from build123d import *

# Parameters (mm, degrees)
SKETCH1_W           = 5.2
SKETCH1_H           = 32
SKETCH1_R           = 1.3
BOSS_EXTRUDE1_DEPTH = 2.8
SKETCH2_W           = 32
SKETCH2_H           = 10
BOSS_EXTRUDE2_DEPTH = 7.9
SKETCH3_W           = 3.95
SKETCH3_H           = 32
CUT_EXTRUDE1_DEPTH  = 7.2
FILLET1_R           = 2


with BuildPart() as part:
    # Sketch1 → Boss-Extrude1 (new body)
    with BuildSketch(Plane(origin=(0, 0, 0), x_dir=(1, 0, 0), z_dir=(0, 1, 0))):
        Rectangle(SKETCH1_W, SKETCH1_H)
        with Locations((0, -8.5)):
            Circle(SKETCH1_R, mode=Mode.SUBTRACT)
        with Locations((0, 8.5)):
            Circle(SKETCH1_R, mode=Mode.SUBTRACT)
    extrude(amount=BOSS_EXTRUDE1_DEPTH)

    # Sketch2 → Boss-Extrude2 (add)
    with BuildSketch(Plane(origin=(2.6, 0, 0), x_dir=(0, 0, -1), z_dir=(1, 0, 0))):
        with Locations((0, 5)):
            Rectangle(SKETCH2_W, SKETCH2_H)
    extrude(amount=BOSS_EXTRUDE2_DEPTH)

    # Sketch3 → Cut-Extrude1 (cut)
    with BuildSketch(Plane(origin=(0, 10, 0), x_dir=(1, 0, 0), z_dir=(0, 1, 0))):
        with Locations((4.575, 0)):
            Rectangle(SKETCH3_W, SKETCH3_H)
    extrude(amount=-CUT_EXTRUDE1_DEPTH, mode=Mode.SUBTRACT)

    # Fillet1
    fillet1_edges = [part.edges().sort_by_distance(p)[0] for p in [
        (6.55, 2.8, 0),
    ]]
    fillet(fillet1_edges, radius=FILLET1_R)


solid = part.part
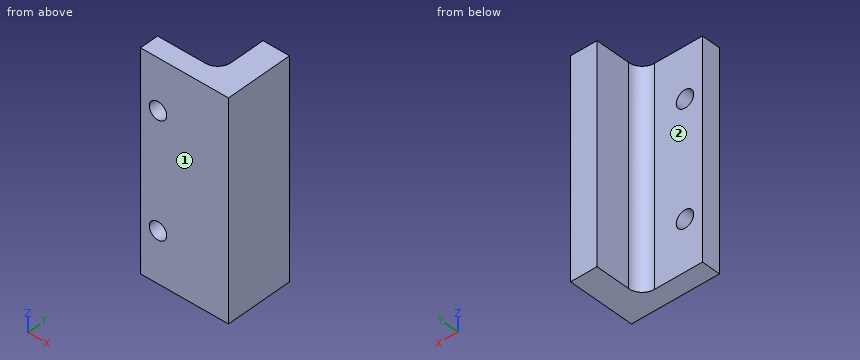
Can you work these out from the model? Positions are in its coordinate system, mm. Face numbers are marked on the shaded views. A direction names the side the tool comes from. Round coordinates to 2 decimals unless told otherwise and drop trailing zeros. Loops run counter-clockwise (first coordinate to the right, second up) from the corner with the lowest first, then second, coordinate; pieces in that order, holes last. Notation, with made-up numbers: (28, 17) - (78, 17) arc R7 ccw to (78, 24) - close; hole circle Ø2 at (-26, -8). An arc over 180 degrees is marked (long way). Write item = value, one per line. Start each with the question number.
(1) For P1, Ø3, axis at y = 9, z = 9.5, coming from the -X side; P2, Ø4, axis at y = 6.5, z = -5.5, coming from the -X side; P3, Ø5, axis at x = 5, z = -9, coming from the +Y side; P4, Ø5.5, axis at x = 2.5, z = -6, coming from the +Y side, each with a flat end and sliding along its axis, tell me the tip position at first contact or that it passes through.
(2) If we section it at D-D (z = -1): Please give me the cut outline in (x, y).
(3) If we section it at C-C (y = 1): Please give me the cut outline in (x, z).
(4) If we section it at B-B (x = 0): Please give me the cut outline in (y, z), and give its area (3 significant figures).
(5) If we section it at A-A (z = 8.5): Please give me the cut outline in (x, y), and give its area (3 significant figures).
(6) If I drill on probe 1 along Z at (x, y) = (0, 1.5); probe 2 along X at (y, z) = (1.6, 8.5); probe 3 along Y at (x, z) = (4.5, 5), over which ranges is the centre line in solid material (lowest first)? Write a range as [from, to].
(7) For the marked faces 1 and 2, which set-ups out of +Z, -Z, +X, -X, +Y, -Y let a thin tool reach every point of the face, with its end or its side?
Ans:
q1.P1 = 6.55
q1.P2 = 6.53
q1.P3 = 10
q1.P4 = 2.93
q2.outline = (-2.6, 0) - (10.5, 0) - (10.5, 10) - (6.55, 10) - (6.55, 4.8) arc R2 cw to (4.55, 2.8) - (-2.6, 2.8) - close
q3.outline = (-2.6, -16) - (10.5, -16) - (10.5, 16) - (-2.6, 16) - close; hole circle Ø2.6 at (0, -8.5); hole circle Ø2.6 at (0, 8.5)
q4.outline = (0, -16) - (2.8, -16) - (2.8, -9.8) - (0, -9.8) - close; (0, -7.2) - (2.8, -7.2) - (2.8, 7.2) - (0, 7.2) - close; (0, 9.8) - (2.8, 9.8) - (2.8, 16) - (0, 16) - close
q4.area = 75.0 mm²
q5.outline = (-2.6, 0) - (-1.3, 0) - (-1.3, 2.8) - (-2.6, 2.8) - close; (1.3, 0) - (10.5, 0) - (10.5, 10) - (6.55, 10) - (6.55, 4.8) arc R2 cw to (4.55, 2.8) - (1.3, 2.8) - close
q5.area = 58.7 mm²
q6.probe_1 = [-16, -9.8], [-7.2, 7.2], [9.8, 16]
q6.probe_2 = [-2.6, -1.3], [1.3, 10.5]
q6.probe_3 = [0, 2.8]
q7.face_1 = +Z, -Z, +X, -X, -Y
q7.face_2 = +Z, -Z, -X, +Y
